```python
from build123d import *

# Parameters (mm, degrees)
BOSS_EXTRUDE3_DEPTH = 28.5
FILLET1_R           = 15
SKETCH8_R           = 9.5
SKETCH8_W           = 8
SKETCH8_H           = 5
CUT_EXTRUDE4_DEPTH  = 10
SKETCH10_R          = 1.75
CUT_EXTRUDE6_DEPTH  = 10
CUT_EXTRUDE9_DEPTH  = 3
SKETCH17_W          = 6
SKETCH17_H          = 2
CUT_EXTRUDE11_DEPTH = 49
FILLET2_R           = 3
CUT_EXTRUDE12_START = -28.5
CUT_EXTRUDE12_DEPTH = 28.5
FILLET3_R           = 5
FILLET4_R           = 5
FILLET5_START       = -1
FILLET5_DEPTH       = 30


with BuildPart() as part:
    # Sketch7 → Boss-Extrude3 (new body)
    with BuildSketch(Plane.XY):
        with BuildLine():
            Line((-75, 0), (75, 0))
            ThreePointArc((75, 0), (82.593171274, 2.949021142), (86.205467416, 10.25))
            Line((86.205467416, 10.25), (84.447221814, 10.25))
            ThreePointArc((84.447221814, 10.25), (65.5, 11.25), (84.447221814, 12.25))
            Line((84.447221814, 12.25), (86.205467416, 12.25))
            ThreePointArc((86.205467416, 12.25), (85.637542957, 14.911308486), (84.447221814, 17.358395861))
            Line((84.447221814, 17.358395861), (84.447221814, 36.5))
            Line((84.447221814, 36.5), (56.447221814, 36.5))
            Line((56.447221814, 36.5), (56.447221814, 10))
            Line((56.447221814, 10), (-56.447221814, 10))
            Line((-56.447221814, 10), (-56.447221814, 36.5))
            Line((-56.447221814, 36.5), (-84.447221814, 36.5))
            Line((-84.447221814, 36.5), (-84.447221814, 17.358395861))
            ThreePointArc((-84.447221814, 17.358395861), (-85.637542957, 14.911308486), (-86.205467416, 12.25))
            Line((-86.205467416, 12.25), (-84.447221814, 12.25))
            ThreePointArc((-84.447221814, 12.25), (-65.5, 11.25), (-84.447221814, 10.25))
            Line((-84.447221814, 10.25), (-86.205467416, 10.25))
            ThreePointArc((-86.205467416, 10.25), (-82.593171274, 2.949021142), (-75, 0))
        make_face()
    extrude(amount=BOSS_EXTRUDE3_DEPTH)

    # Fillet1
    fillet1_edges = [part.edges().sort_by_distance(p)[0] for p in [
        (-56.447221814, 10, 14.25),
        (56.447221814, 10, 14.25),
    ]]
    fillet(fillet1_edges, radius=FILLET1_R)

    # Sketch8 → Cut-Extrude4 (cut)
    with BuildSketch(Plane(origin=(0, 10, 0), x_dir=(1, 0, 0), z_dir=(0, 1, 0))):
        with Locations(Location((21, -14.25, 0), (0, 0, 270))):
            Circle(SKETCH8_R)
        with Locations(Location((-21, -14.25, 0), (0, 0, 270))):
            Circle(SKETCH8_R)
        with Locations((0, -14.25)):
            Rectangle(SKETCH8_W, SKETCH8_H)
    extrude(amount=-CUT_EXTRUDE4_DEPTH, mode=Mode.SUBTRACT)

    # Sketch10 → Cut-Extrude6 (cut)
    with BuildSketch(Plane(origin=(0, 36.5, 0), x_dir=(1, 0, 0), z_dir=(0, 1, 0))):
        with Locations(Location((70.447221814, -14.25, 0), (0, 0, 180))):
            Circle(SKETCH10_R)
        with Locations(Location((-70.447221814, -14.25, 0), (0, 0, 180))):
            Circle(SKETCH10_R)
    extrude(amount=-CUT_EXTRUDE6_DEPTH, mode=Mode.SUBTRACT)

    # Sketch13 → Cut-Extrude9 (cut)
    with BuildSketch(Plane(origin=(0, 36.5, 0), x_dir=(1, 0, 0), z_dir=(0, 1, 0))):
        Polygon((67.697221814, -12.66228676), (67.697221814, -15.83771324), (70.447221814, -17.425426481), (73.197221814, -15.83771324), (73.197221814, -12.66228676), (70.447221814, -11.074573519), align=None)
        Polygon((-70.447221814, -17.425426481), (-67.697221814, -15.83771324), (-67.697221814, -12.66228676), (-70.447221814, -11.074573519), (-73.197221814, -12.66228676), (-73.197221814, -15.83771324), align=None)
    extrude(amount=-CUT_EXTRUDE9_DEPTH, mode=Mode.SUBTRACT)

    # Sketch17 → Cut-Revolve1 (revolve, cut)
    with BuildSketch(Plane.ZY.offset(-75)):
        with Locations((22, 23.75)):
            Rectangle(SKETCH17_W, SKETCH17_H)
        with Locations((6.5, 23.75)):
            Rectangle(SKETCH17_W, SKETCH17_H)
    cut_revolve1 = revolve(axis=Axis((75, 11.25, 28.5), (0, 0, -1)), mode=Mode.SUBTRACT)

    # Mirror1: Cut-Revolve1 across plane
    add(cut_revolve1.mirror(Plane(origin=(0, 0, 0), x_dir=(0, 0, 1), z_dir=(1, 0, 0))), mode=Mode.SUBTRACT)

    # Sketch18 → Cut-Extrude11 (cut)
    with BuildSketch(Plane.XY.offset(28.5)):
        Polygon((-75, 11.25), (-65.964963095, 8.314338553), (-65.964963095, 0), (-86.964963095, 0), (-86.964963095, 11.25), align=None)
        Polygon((86.964963095, 11.25), (75, 11.25), (65.964963095, 8.314338553), (65.964963095, 0), (86.964963095, 0), align=None)
    extrude(amount=-CUT_EXTRUDE11_DEPTH, mode=Mode.SUBTRACT)

    # Fillet2
    # the kernel refuses this fillet: 3 mm, written as the material it takes off along each edge
    with BuildSketch(Plane(origin=(-65.964963095, 0, 36), x_dir=(1, 0, 0), z_dir=(0, 0, -1)), Plane(origin=(65.964963095, 0, 36), x_dir=(0, 1, 0), z_dir=(0, 0, -1))) as fillet2_piece_1:
        with BuildLine():
            CenterArc((FILLET2_R, -FILLET2_R), FILLET2_R, 90, 90)
            Line((0, -FILLET2_R), (0, 0))
            Line((0, 0), (FILLET2_R, 0))
        make_face()
    extrude(amount=43.5, mode=Mode.SUBTRACT)

    # Sketch20 → Cut-Extrude12 (cut)
    with BuildSketch(Plane.XY.offset(28.5).offset(CUT_EXTRUDE12_START)):
        with BuildLine():
            Line((57.587719851, 5), (-57.587719851, 5))
            ThreePointArc((-57.587719851, 5), (-58.757162737, 2.39447982), (-60.313696857, 0))
            Line((-60.313696857, 0), (60.313696857, 0))
            ThreePointArc((60.313696857, 0), (58.757162737, 2.39447982), (57.587719851, 5))
        make_face()
    extrude(amount=CUT_EXTRUDE12_DEPTH, mode=Mode.SUBTRACT)

    # Fillet3
    # the kernel refuses this fillet: 5 mm, written as the material it takes off along each edge
    with BuildSketch(Plane(origin=(-60.313696857, 0, -7.959028746), x_dir=(0.5375468252695589, 0.8432339003162873, 0), z_dir=(0, 0, 1))) as fillet3_piece_1:
        with BuildLine():
            CenterArc((2.753393728, 4.981456882), FILLET3_R, 213.309669326, 61.62636665)
            Line((-1.425179749, 2.235637571), (-1.508751219, 2.180721184))
            ThreePointArc((-1.508751219, 2.180721184), (-0.796913265, 1.064064103), (-0.08432339, -0.053754683))
            Line((-0.08432339, -0.053754683), (-0.008604355, -0.099629138))
            ThreePointArc((-0.008604355, -0.099629138), (1.591805749, -0.168609535), (3.192215854, -0.099629138))
            Line((3.192215854, -0.099629138), (3.183611498, 0))
        make_face()
    extrude(amount=44.418057492, mode=Mode.SUBTRACT)

    # Fillet4
    fillet4_edges = [part.edges().sort_by_distance(p)[0] for p in [
        (-57.587719851, 5, 14.25),
        (57.587719851, 5, 14.25),
    ]]
    fillet(fillet4_edges, radius=FILLET4_R)

    # Fillet5: read off the stored shape, not the designer's step
    # Fillet5 outline → Fillet5 (cut)
    with BuildSketch(Plane.XY.offset(FILLET5_START)):
        with BuildLine():
            ThreePointArc((62.964963095, 0), (60.500818254, 0.685449294), (58.69804707, 2.499799478))
            ThreePointArc((58.69804707, 2.499799478), (58.728163344, 2.446889634), (58.757633161, 2.393617021))
            ThreePointArc((58.757633161, 2.393617021), (59.489422728, 1.16674692), (60.313696857, 0))
            Line((60.313696857, 0), (62.964963095, 0))
        make_face()
    extrude(amount=FILLET5_DEPTH, mode=Mode.SUBTRACT)


solid = part.part
```
Model file for the job. Use its own axes, mm. A direction names the side the tool comes from. Give positions to 0.01 mm unless a question says otherwise; leave off trailing zeros. Loops run counter-clockwise (first coordinate to the right, second up) from the corner with the lowest first, then second, coordinate; pieces in that order, holes last. Notation, with made-up numbers: M 80,39.25 L 88,39.25 A30 cw 88,68.25 Z; hole C 23,70 d7. An arc over 180 degrees is marked long. Use one line per item in the form item = value.
Item 1: Two-plate mould, pull along X, no slides. Class faces 4 (the flat face through (65.965, 6, 14)), 5 (the flat face through (0, 9, 28.5)), 6 (the flat face through (67, 20, 25)): released by +X, released by -X, zero draft, split by the parting line, or undercut.
Filled in:
face_4 = released by +X
face_5 = zero draft
face_6 = undercut
Item 2: Which spindle directions (+Z, -Z, +X, -X, +Y, -Y) get a long thin tool onto all of the face, cutting with end or side? Do faces 1 (the flat face through (56.447, 31, 14)), 2 (the cylindrical face through (-67.955, 20.34, 22.042)), 3 (the flat face through (-73.197, 35, 14)). Say none if no direction does.
Filled in:
face_1 = +Z, -Z, +Y
face_2 = none
face_3 = +Y
Item 3: Slice it at B-B on y = 31.5. List the corners of the cut face in (x, z), and give its area (3 significant figures).
Filled in:
outline = M -84.45,0 L -56.45,0 L -56.45,28.5 L -84.45,28.5 Z; M 56.45,0 L 84.45,0 L 84.45,28.5 L 56.45,28.5 Z; hole C -70.45,14.25 d3.5; hole C 70.45,14.25 d3.5
area = 1,580 mm^2
Item 4: Slice it at A-A on x = 21. List the corners of the cut face in (y, z).
Filled in:
outline = M 5,0 L 10,0 L 10,4.75 L 5,4.75 Z; M 5,23.75 L 10,23.75 L 10,28.5 L 5,28.5 Z
Item 5: Drill centre lines: L1, parallel to Y at x = 75, z = 19.5; L2, parallel to X at y = 18.5, z = 10.5; L3, parallel to X at y = 11.25, z = 6.75. Where is each one in solid material? Low to high.
Filled in:
L1 = 20.75 to 22.75, 24.75 to 36.5
L2 = -84.45 to -81.14, -68.86 to -54.97, 54.97 to 68.86, 81.14 to 84.45
L3 = -65.5 to -63.5, -61.5 to -47.44, 47.44 to 61.5, 63.5 to 65.5
Item 6: Slice it at C-C on x = 75. List the corners of the cut face in (y, z), and give its area (3 significant figures).
Filled in:
outline = M 20.75,0 L 36.5,0 L 36.5,28.5 L 20.75,28.5 Z; hole M 22.75,3.5 L 24.75,3.5 L 24.75,9.5 L 22.75,9.5 Z; hole M 22.75,19 L 24.75,19 L 24.75,25 L 22.75,25 Z
area = 425 mm^2
Item 7: Flat gauge pins, fed straight in: pin 1 Ø3 at (x, z) = (-71, 14.5) entering from +Y; pin 2 Ø3 at (x, z) = (70.45, 14.25) entering from +Y; pin 3 Ø8.5 at (x, z) = (8, 8.5) entering from -Y; pin 4 Ø8.5 at (x, z) = (-18.5, 15.5) entering from +Y. Where does each tip first touch, or does it go through?
Filled in:
pin_1 = 33.5
pin_2 = 26.5
pin_3 = 5
pin_4 = through
Item 8: Slice it at D-D on z = 14.25. Give the number of separate pieces and of enclosed holes in the cut face, and give its area (3 significant figures).
Filled in:
separate_pieces = 4
enclosed_holes = 0
area = 1,680 mm^2
